```python
from build123d import *

# Parameters (mm, degrees)
BOSS_EXTRUDE1_DEPTH = 50.8


with BuildPart() as part:
    # Sketch1 → Boss-Extrude1 (new body)
    with BuildSketch(Plane(origin=(0, 0, 0), x_dir=(1, 0, 0), z_dir=(0, 1, 0))):
        Polygon((2.749630657, -1.5875), (0, 0), (0, -26.250738686), (3.175, -26.250738686), (3.175, -0.850738686), align=None)
        Polygon((15.875, 21.14630657), (13.125369343, 22.73380657), (0, 0), (3.175, 0), (3.175, -0.850738686), align=None)
        Polygon((3.175, 0), (0, 0), (2.749630657, -1.5875), (3.175, -0.850738686), align=None)
    extrude(amount=BOSS_EXTRUDE1_DEPTH)


solid = part.part
```
Geometry check sheet. Reference: the model listing, model coordinates, mm. A direction names the side the tool comes from. Round coordinates to 2 decimals unless told otherwise and drop trailing zeros. Loops run counter-clockwise (first coordinate to the right, second up) from the corner with the lowest first, then second, coordinate; pieces in that order, holes last. Notation, with made-up numbers: M -20,15.25 L 35,15.25 A29 cw 35,47.25 Z; hole C 86.5,67.25 d10. An arc over 180 degrees is marked long. Return JSON: item names as keys, results as strings. Group by question number.
(1) Set-up check for faces 1 (the face through (3.175, 25, 14)), 2 (the face through (3, 50.8, 2)): record each of +Z, -Z, +X, -X, +Y, -Y from which the full face is reachable in a straight line by a thin tool's end or side.
(2) Section check C-C, the plane x = 8.75. Enter the section's corners in (y, z), and give its area (3 significant figures).
(3) Section check A-A, the plane y = 43.5. Enter the section's corners in (x, z) (3 decimals), and give its area (3 significant figures).
(4) Section check B-B, the plane z = 4.5. Enter the section's corners in (x, y) (3 decimals).
(5) Go/stop test with flat-tipped pins: pin 1 (5 mm diameter, centred on x = 12.5, y = 8, fed in from +Z); pin 2 (1.5 mm diameter, centred on x = 8, y = 45.5, fed in from -Z); pin 3 (5 mm diameter, centred on x = 4, y = 21.5, fed in from +Z). Record where each tip stops, or that it passes through.
(6) Scan lines: line 1 along X through (y, z) = (34.5, 11) (3 decimals); line 2 along Z through (x, y) = (7, 2); line 3 along Z through (x, y) = (14.25, 26). Record each from-to range of solid material in increasing order. Write a range as [from, to].
Data:
{
 "1": {"face 1": "+Z, +X, +Y, -Y", "face 2": "+Z, -Z, +X, -X, +Y"},
 "2": {"outline": "M 0,-15.16 L 50.8,-15.16 L 50.8,-8.81 L 0,-8.81 Z", "area": "323 mm²"},
 "3": {"outline": "M 0,0 L 13.125,-22.734 L 15.875,-21.146 L 3.175,0.851 L 3.175,26.251 L 0,26.251 Z", "area": "164 mm²"},
 "4": {"outline": "M 0,0 L 3.175,0 L 3.175,50.8 L 0,50.8 Z"},
 "5": {"pin 1": "z = -10.97", "pin 2": "z = -15.16", "pin 3": "z = 26.25"},
 "6": {"line 1": "[0, 3.175]", "line 2": "[-12.12, -5.77]", "line 3": "[-22.08, -18.33]"}
}
